from build123d import *

# Parameters (mm, degrees)
PAD_DEPTH = 15
FILLET_R  = 1


with BuildPart() as part:
    # Sketch → Pad (new body)
    with BuildSketch(Plane.XY):
        Polygon((0, -10), (40, -10), (40, -26), (0, -26), (0, -66), (50, -66), (50, -46), (45, -46), (45, -56), (10, -56), (10, -36), (50, -36), (50, 0), (0, 0), align=None)
    extrude(amount=PAD_DEPTH)

    # Fillet
    fillet_edges = [part.edges().sort_by_distance(p)[0] for p in [
        (50, -46, 7.5),
        (45, -46, 7.5),
    ]]
    fillet(fillet_edges, radius=FILLET_R)


solid = part.part
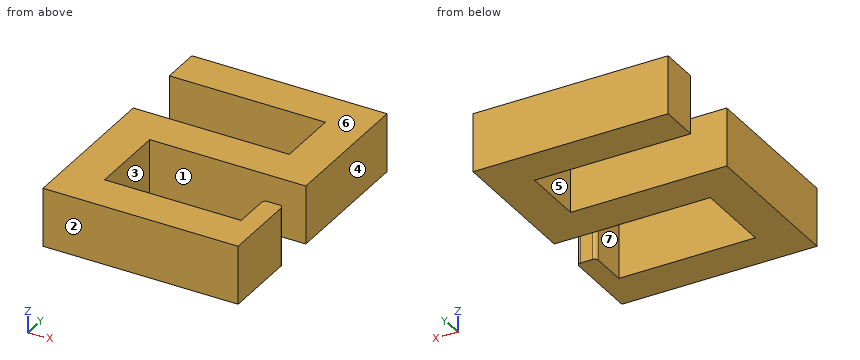
Could you check a few things on this model? Use its own coordinates, in mm. Face numbers are marked on the shaded views. A direction names the side the tool comes from. Give positions to 0.01 mm unless a question says otherwise; leave off trailing zeros. Write each loop counter-clockwise with the first axis right and the second up, starting at its lowest first coordinate (ties: lowest second). Pieces come first, ordered by that corner, then holes. Notation, with made-up numbers: (4, 75) - (55, 75) arc R31 ccw to (55, 111) - close; hole circle Ø4 at (20, 24). An arc over 180 degrees is marked (long way). Use CSV: the item, a comma, the result in double quotes. Start each with the question number.
Item 1: I want a section at A-A, the plane y = -48. Please give me the cut outline in (x, z), then the cut area to 3 significant figures.
Item 2: I want a section at C-C, the plane z = 8.75. Please give me the cut outline in (x, y).
Item 3: I want a section at B-B, the plane x = 32. Please give me the cut outline in (y, z).
Item 4: If we mould it in two halves opening along Y, with no side actions, what happens to the marked faces 1, 2, 3 and 4? For each: pulls with the +Y half, pulls with the -Y half, needs draft (parallel to the pull), parting line crosses it, or undercut.
Item 5: I want a section at D-D, the plane x = 3.5. Please give me the cut outline in (y, z).
Item 6: If I drill on line 1 along Y through (x, z) = (35.5, 13); line 2 along Y through (x, z) = (46, 5); line 3 along X through (y, z) = (-14, 7.5), over which ranges is the centre line in solid material (lowest first)?
Item 7: For the marked faces 5, 6 and 7, which set-ups out of +Z, -Z, +X, -X, +Y, -Y let a thin tool reach every point of the face, with its end or its side?
Findings:
1,outline,"(0, 0) - (10, 0) - (10, 15) - (0, 15) - close; (45, 0) - (50, 0) - (50, 15) - (45, 15) - close"
1,area,"225 mm2"
2,outline,"(0, -66) - (50, -66) - (50, -47) arc R1 ccw to (49, -46) - (46, -46) arc R1 ccw to (45, -47) - (45, -56) - (10, -56) - (10, -36) - (50, -36) - (50, 0) - (0, 0) - (0, -10) - (40, -10) - (40, -26) - (0, -26) - close"
3,outline,"(-66, 0) - (-56, 0) - (-56, 15) - (-66, 15) - close; (-36, 0) - (-26, 0) - (-26, 15) - (-36, 15) - close; (-10, 0) - (0, 0) - (0, 15) - (-10, 15) - close"
4,face 1,"undercut"
4,face 2,"pulls with the -Y half"
4,face 3,"undercut"
4,face 4,"needs draft"
5,outline,"(-66, 0) - (-26, 0) - (-26, 15) - (-66, 15) - close; (-10, 0) - (0, 0) - (0, 15) - (-10, 15) - close"
6,line 1,"y = -66 to -56, -36 to -26, -10 to 0"
6,line 2,"y = -66 to -46, -36 to 0"
6,line 3,"x = 40 to 50"
7,face 5,"+Z, -Z, -X"
7,face 6,"+Z, +X, -X, +Y, -Y"
7,face 7,"+Z, -Z"
